Geometry: final body of the model. Coordinates: model frame, mm. Give positions to 0.01 mm unless a question says otherwise; leave off trailing zeros. Write each loop counter-clockwise with the first axis right and the second up, starting at its lowest first coordinate (ties: lowest second). Pieces come first, ordered by that corner, then holes. Notation, with made-up numbers: (73.25, 45) -> (95.25, 45) arc R16 cw to (95.25, 52) -> close; hole circle Ø7 at (3.5, 85.5). An arc over 180 degrees is marked (long way). Use CSV: the item, a comma, the result in double quotes. Start each with the question number.
1) Section C-C (x = -10). Output: boundary loops of the cut face in (y, z).
2) Section A-A (x = 16). Output: boundary loops of the cut face in (y, z).
3) Section B-B (z = 10). Output: boundary loops of the cut face in (x, y), plus the area to 3 significant figures.
4) Material intervals for line 1 (Y direction, x = -16, z = -10), sorted ascending. Write a range as [from, to].
5) Contact query for flat-ended pins moving along their axis: P1, Ø0.8, axis at x = 9.5, y = 2.5, coming from the +Z side; P2, Ø0.8, axis at y = 2, z = -10, coming from the -X side; P3, Ø2, axis at x = -10, y = 2.5, coming from the -Z side. Output: stop coordinate, or through.
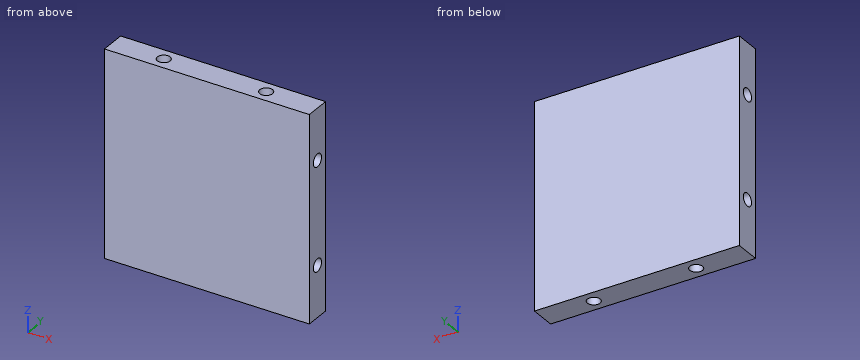
```python
from build123d import *

# Parameters (mm, degrees)
SKETCH1_W           = 40
SKETCH1_H           = 40
BOSS_EXTRUDE1_DEPTH = 5
SKETCH2_R           = 1.25
CUT_EXTRUDE1_DEPTH  = 5
CIRPATTERN1_COUNT   = 4


with BuildPart() as part:
    # Sketch1 → Boss-Extrude1 (new body)
    with BuildSketch(Plane(origin=(0, 0, 0), x_dir=(1, 0, 0), z_dir=(0, 1, 0))):
        Rectangle(SKETCH1_W, SKETCH1_H)
    extrude(amount=BOSS_EXTRUDE1_DEPTH)

    # Sketch2 → Cut-Extrude1 (cut)
    with BuildSketch(Plane.XY.offset(20)):
        with Locations((-10, 2.5)):
            Circle(SKETCH2_R)
        with Locations(Location((10, 2.5, 0), (0, 0, 180))):
            Circle(SKETCH2_R)
    cut_extrude1 = extrude(amount=-CUT_EXTRUDE1_DEPTH, mode=Mode.SUBTRACT)

    # CirPattern1: Cut-Extrude1 ×4 about axis
    cirpattern1_axis = Axis((0, 0, 0), (0, 1, 0))
    for i in range(1, CIRPATTERN1_COUNT):
        add(cut_extrude1.rotate(cirpattern1_axis, i * 360 / CIRPATTERN1_COUNT), mode=Mode.SUBTRACT)


solid = part.part
```
Answers follow:
1,outline,"(0, -20) -> (1.25, -20) -> (1.25, -15) -> (3.75, -15) -> (3.75, -20) -> (5, -20) -> (5, 20) -> (3.75, 20) -> (3.75, 15) -> (1.25, 15) -> (1.25, 20) -> (0, 20) -> close"
2,outline,"(0, -20) -> (5, -20) -> (5, 20) -> (0, 20) -> close; hole circle Ø2.5 at (2.5, -10); hole circle Ø2.5 at (2.5, 10)"
3,outline,"(-20, 0) -> (20, 0) -> (20, 1.25) -> (15, 1.25) -> (15, 3.75) -> (20, 3.75) -> (20, 5) -> (-20, 5) -> (-20, 3.75) -> (-15, 3.75) -> (-15, 1.25) -> (-20, 1.25) -> close"
3,area,"175 mm^2"
4,line 1,"y = [0, 1.25], [3.75, 5]"
5,P1,"stops at z = 15"
5,P2,"stops at x = -15"
5,P3,"stops at z = -15"
